from build123d import *

# Parameters (mm, degrees)
F0_W     = 20
F0_H     = 94
F1_DEPTH = 25
F2_R     = 5
F2_R_2   = 4
F3_DEPTH = 17
F4_DEPTH = 20
F5_START = -16
F5_DEPTH = 1
F6_R     = 5
F7_R     = 2
F8_DEPTH = 3


# Not quite as in the source:
# - a pattern or mirror of a feature is missing from the dataset's text; its kind, count and spacing are read off the source's solid


with BuildPart() as f1:
    # F0 (on Top) → F1 (new body)
    with BuildSketch(Plane.XY):
        with Locations((-55, 0)):
            Rectangle(F0_W, F0_H)
    extrude(amount=F1_DEPTH)

    # F2 (on face) → F3 (cut)
    with BuildSketch(Plane.YZ.offset(-45)):
        with BuildLine():
            Line((-32.4501655647, 25), (-47, 25))
            Line((-47, 25), (-47, 8.5147186258))
            ThreePointArc((-47, 8.5147186258), (-35.3095842402, 7.0501256289), (-29, 17))
            ThreePointArc((-29, 17), (-29.8993025293, 21.3561348241), (-32.4501655647, 25))
        make_face()
        with Locations((-40, 17)):
            Circle(F2_R, mode=Mode.SUBTRACT)
        with BuildLine():
            Line((-29.753049234, 25), (-32.4501655647, 25))
            ThreePointArc((-32.4501655647, 25), (-29.8993025293, 21.3561348241), (-29, 17))
            ThreePointArc((-29, 17), (-35.3095842402, 7.0501256289), (-47, 8.5147186258))
            Line((-47, 8.5147186258), (-47, 6.0455488499))
            ThreePointArc((-47, 6.0455488499), (-33.7550020016, 5.598245749), (-27, 17))
            ThreePointArc((-27, 17), (-27.7075153049, 21.2302269468), (-29.753049234, 25))
        make_face()
        with BuildLine():
            Line((47, 25), (-29.753049234, 25))
            ThreePointArc((-29.753049234, 25), (-27.7075153049, 21.2302269468), (-27, 17))
            ThreePointArc((-27, 17), (-33.7550020016, 5.598245749), (-47, 6.0455488499))
            Line((-47, 6.0455488499), (-47, 3))
            Line((-47, 3), (47, 3))
            Line((47, 3), (47, 25))
        make_face()
        with Locations((-40, 17)):
            Circle(F2_R)
        with Locations((-40, 17)):
            Circle(F2_R_2, mode=Mode.SUBTRACT)
    extrude(amount=-F3_DEPTH, mode=Mode.SUBTRACT)

    # F2 (on face) → F4 (cut, through all)
    with BuildSketch(Plane.YZ.offset(-45)):
        with Locations((-40, 17)):
            Circle(F2_R_2)
    f4 = extrude(amount=-F4_DEPTH, mode=Mode.SUBTRACT)

    # F4_copies: F4 across plane
    add(f4.mirror(Plane.ZX), mode=Mode.SUBTRACT)

    # F2 (on face) → F5 (join)
    with BuildSketch(Plane.YZ.offset(-45).offset(F5_START)):
        with Locations((-40, 17)):
            Circle(F2_R)
        with Locations((-40, 17)):
            Circle(F2_R_2, mode=Mode.SUBTRACT)
    f5 = extrude(amount=-F5_DEPTH)

    # F5_copies: F5 across plane
    add(f5.mirror(Plane.ZX))

    # F6
    f6_edges = [f1.edges().sort_by_distance(p)[0] for p in [
        (-63.5, -47, 25),
        (-63.5, 47, 25),
    ]]
    fillet(f6_edges, radius=F6_R)

    # F7 (on face) → F8 (cut, through all)
    with BuildSketch(Plane.XY.offset(3)):
        with Locations((-53.5, 0)):
            Circle(F7_R)
    extrude(amount=-F8_DEPTH, mode=Mode.SUBTRACT)


solid = f1.part
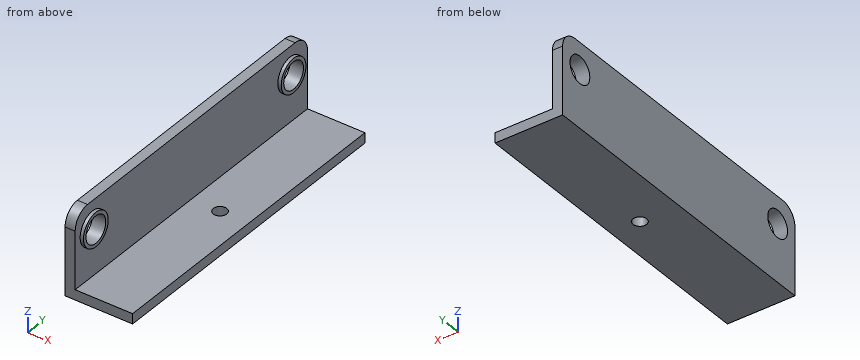
Here's how the part is built. I have some questions about the finished solid (model axes, mm). Round coordinates to 2 decimals unless told otherwise and drop trailing zeros. Order: outer loops, then holes, each group sorted by start corner. A loop starts at its lowest first (then second) coordinate and runs counter-clockwise, first axis right, second up. Notation, with made-up numbers: (12.5, 55) -> (43.5, 55) arc R24 cw to (43.5, 89) -> close; hole circle Ø9 at (89, 72). An arc over 180 degrees is marked (long way). Return JSON: item names as keys, results as strings.
Q1. If we section it at B-B on z = 17: List the corners of the cut face in (x, y) for me, plus the area to 3 significant figures.
Filled sheet:
{"outline": "(-65, -47) -> (-62, -47) -> (-62, -45) -> (-61, -45) -> (-61, -44) -> (-65, -44) -> close; (-65, -36) -> (-61, -36) -> (-61, -35) -> (-62, -35) -> (-62, 35) -> (-61, 35) -> (-61, 36) -> (-65, 36) -> close; (-65, 44) -> (-61, 44) -> (-61, 45) -> (-62, 45) -> (-62, 47) -> (-65, 47) -> close", "area": "238 mm^2"}
Q2. If we section it at A-A on x = -53.5: List the corners of the cut face in (y, z) for me.
Filled sheet:
{"outline": "(-47, 0) -> (-2, 0) -> (-2, 3) -> (-47, 3) -> close; (2, 0) -> (47, 0) -> (47, 3) -> (2, 3) -> close"}
Q3. If we section it at D-D on y = 0: List the corners of the cut face in (x, z) for me.
Filled sheet:
{"outline": "(-65, 0) -> (-55.5, 0) -> (-55.5, 3) -> (-62, 3) -> (-62, 25) -> (-65, 25) -> close; (-51.5, 0) -> (-45, 0) -> (-45, 3) -> (-51.5, 3) -> close"}
Q4. I need wall thicknesses on line 1 along Y through (x, z) = (-53.5, 2); line 2 along Z through (x, y) = (-62.5, 40); line 3 along Z through (x, y) = (-59.5, 41.5). Which ranges of each line are inside material? Lowest first, please. Write a range as from..to.
Filled sheet:
{"line 1": "y = -47..-2, 2..47", "line 2": "z = 0..13, 21..25", "line 3": "z = 0..3"}
Q5. If we section it at C-C on y = 40: List the corners of the cut face in (x, z) for me.
Filled sheet:
{"outline": "(-65, 0) -> (-45, 0) -> (-45, 3) -> (-62, 3) -> (-62, 12) -> (-61, 12) -> (-61, 13) -> (-65, 13) -> close; (-65, 21) -> (-61, 21) -> (-61, 22) -> (-62, 22) -> (-62, 25) -> (-65, 25) -> close"}
Q6. For pin 1 Ø6.5 at (y, z) = (-40, 17) entering from +X; pin 2 Ø3 at (x, y) = (-50.5, 34) entering from +Z; pin 3 Ø11 at (y, z) = (41, 18) entering from +X; pin 4 Ø11 at (y, z) = (-17.5, 14) entering from +X, each with a flat end and sliding along its axis, tell me the tip position at first contact or that it passes through.
Filled sheet:
{"pin 1": "passes through", "pin 2": "stops at z = 3", "pin 3": "stops at x = -61", "pin 4": "stops at x = -62"}
